Here's how the part is built. I have some questions about the finished solid (model axes, mm). A direction names the side the tool comes from. Give positions to 0.01 mm unless a question says otherwise; leave off trailing zeros. Order: outer loops, then holes, each group sorted by start corner. A loop starts at its lowest first (then second) coordinate and runs counter-clockwise, first axis right, second up.
from build123d import *

# Parameters (mm, degrees)
BOSS_EXTRUDE1_DEPTH = 850
SKETCH2_W           = 829.503147771
SKETCH2_H           = 24.520289532
CUT_EXTRUDE1_DEPTH  = 20


with BuildPart() as part:
    # Sketch1 → Boss-Extrude1 (new body)
    with BuildSketch(Plane(origin=(0, 0, 0), x_dir=(0, 0, -1), z_dir=(1, 0, 0))):
        with BuildLine():
            Line((-147.74064655, -92.809040889), (21.737933493, 88.875862637))
            add(Edge.make_bspline(
                [(21.737933493, 88.875862637), (22.846353546, 90.074456327), (23.208127069, 91.669385546)],
                knots=[0, 0, 0, 1, 1, 1], degree=2))
            Line((23.208127069, 91.669385546), (28.470152179, 115.618408292))
            ThreePointArc((28.470152179, 115.618408292), (32.569812262, 122.282745924), (40.094456308, 124.427586441))
            ThreePointArc((40.094456308, 124.427586441), (81.491387891, 105.200191819), (109.979351041, 69.537401631))
            ThreePointArc((109.979351041, 69.537401631), (110.794083493, 64.647138854), (109.33864767, 59.907923142))
            Line((109.33864767, 59.907923142), (99.458915624, 47.413226279))
            Line((99.458915624, 47.413226279), (20.929242749, -73.511865602))
            ThreePointArc((20.929242749, -73.511865602), (19.968049413, -75.596855125), (19.638607292, -77.868977882))
            ThreePointArc((19.638607292, -77.868977882), (-64.487922257, -80.444221731), (-147.74064655, -92.809040889))
        make_face()
    extrude(amount=BOSS_EXTRUDE1_DEPTH)

    # Sketch2 → Cut-Extrude1 (cut)
    with BuildSketch(Plane(origin=(0, -0.642785482, -2.925505639), x_dir=(1, 0, 0), z_dir=(0, 0.21459881636528488, 0.9767022821794873))):
        with Locations((424.628691519, 106.774279434)):
            Rectangle(SKETCH2_W, SKETCH2_H)
    extrude(amount=-CUT_EXTRUDE1_DEPTH, mode=Mode.SUBTRACT)


solid = part.part
Q1. If we section it at B-B on z = -88.5: List the corners of the cut face in (x, y) for me, plus the area to 3 significant figures.
Filled sheet:
outline: (0, 30.54) - (850, 30.54) - (850, 99.15) - (0, 99.15) - close
area: 58,300 mm2
Q2. If we section it at A-A on y = -30.5: List the corners of the cut face in (x, z) for me, plus the area to 3 significant figures.
Filled sheet:
outline: (0, -48.86) - (850, -48.86) - (850, 89.62) - (0, 89.62) - close
area: 118,000 mm2
Q3. For faces 4 (the face through (418.82, 99.52, -45.41)), 5 (the face through (418.822, 113.502, -38.1)), 6 (the face through (0, -7, -12)), which set-ups out of +Z, -Z, +X, -X, +Y, -Y let a thin tool reach every point of the face, with its end or its side?
Filled sheet:
face 4: none
face 5: +Z
face 6: +Z, -Z, -X, +Y, -Y
Q4. I need wall thicknesses on L1, parallel to Y at x = 495, z = -82.5; L2, parallel to Z at x = 774, y = -14; L3, parallel to Y at x = 810, z = 56. Which ranges of each line are inside material? Lowest first, please.
Filled sheet:
L1: y = 21.3 to 104.4
L2: z = -59.58 to 74.23
L3: y = -79.74 to 5.54
Q5. I'm going to push flat-ended pins straight in: P1, Ø12, axis at x = 315.5, y = 75.5, coming from the +Z side; P2, Ø6, axis at x = 197.5, z = 121, coming from the -Y side; P3, Ø6, axis at x = 463.5, y = 73.5, coming from the +Z side. Where does each tip first touch, or does it pass through?
Filled sheet:
P1: stops at z = -3.66
P2: stops at y = -88.27
P3: stops at z = -4.6
Q6. Thinking about a two-plate mould opening in Z: for faces 1 (the face through (419.05, -3.24, 64.19)), 2 (the face through (418.822, 89.553, -32.838)), 3 (the face through (850, -7, -12)), which applies, released by +Z, released by -Z, zero draft, split by the parting line, or undercut?
Filled sheet:
face 1: released by +Z
face 2: undercut
face 3: zero draft
